The model under review builds one solid part; all positions refer to its coordinate system, in mm. A direction names the side the tool comes from. Coordinates: 2 decimals unless noted, no trailing zeros. Write each loop counter-clockwise with the first axis right and the second up, starting at its lowest first coordinate (ties: lowest second). Pieces come first, ordered by that corner, then holes. Notation, with made-up numbers: (74, 30.25) - (88, 30.25) arc R26 ccw to (88, 60.25) - close; hole circle Ø6 at (-13.75, -11.75). An arc over 180 degrees is marked (long way). Answer as CSV lines item,"result". Start each with the question number.
```python
from build123d import *

# Parameters (mm, degrees)
BOSS_EXTRUDE1_OUTLINE_R = 1.1
BOSS_EXTRUDE1_DEPTH     = 3
BOSS_EXTRUDE2_DEPTH     = 11
BOSS_EXTRUDE3_REACH     = 87.92
SKETCH5_W               = 5
SKETCH5_H               = 2


# Read off the part's stored shape, not the designer's step: Boss-Extrude1
with BuildPart() as part:
    # Boss-Extrude1 outline → Boss-Extrude1 (new body)
    with BuildSketch(Plane.XY):
        with BuildLine():
            Line((-16.861546239, -6.996941033), (-16.235942246, -6.960409413))
            ThreePointArc((-16.235942246, -6.960409413), (-14.264395542, -6.327834493), (-12.678246106, -4.996941033))
            ThreePointArc((-12.678246106, -4.996941033), (13.21501224, 8.679812005), (42.365911354, 5.89781951))
            Line((42.365911354, 5.89781951), (60.907203246, -17.149637471))
            Line((60.907203246, -17.149637471), (78.805808552, -2.750510239))
            Line((78.805808552, -2.750510239), (58.935546262, 21.948902186))
            Line((58.935546262, 21.948902186), (48.942403416, 13.909586673))
            ThreePointArc((48.942403416, 13.909586673), (12.120494673, 18.357071745), (-21.044846371, 1.753058967))
            ThreePointArc((-21.044846371, 1.753058967), (-21.710837424, -3.940345657), (-16.861546239, -6.996941033))
        make_face()
        Polygon((-15.008213446, -0.217369118), (-15.079375496, -0.657391661), (-14.639590345, -0.883380518), (-14.841297197, -1.275911723), (-14.495267888, -1.621941033), (-14.810453449, -1.937126594), (-14.586057014, -2.377726392), (-14.983250587, -2.580016139), (-14.906078059, -3.068407726), (-15.346355155, -3.137977509), (-15.423969348, -3.626299102), (-15.864183346, -3.556331166), (-16.088978162, -3.996727842), (-16.485988624, -3.794078961), (-16.835934444, -4.143392379), (-17.150834826, -3.827921897), (-17.591637385, -4.051919766), (-17.793567832, -3.654543407), (-18.282029013, -3.731274208), (-18.351200586, -3.290934374), (-18.839451787, -3.212878581), (-18.769085755, -2.772728041), (-19.209278949, -2.547535028), (-19.006271099, -2.150708001), (-19.355267888, -1.800446409), (-19.039512742, -1.485831463), (-19.263111863, -1.044826504), (-18.865553043, -0.843255522), (-18.941842054, -0.354725146), (-18.501439842, -0.285951839), (-18.422942512, 0.202228569), (-17.982855791, 0.131464499), (-17.757264764, 0.571453851), (-17.360621498, 0.368087198), (-17.01004442, 0.716767072), (-16.695715168, 0.400727521), (-16.254508168, 0.623927711), (-16.053296817, 0.226186755), (-15.564697645, 0.302033914), (-15.496322662, -0.138430316), align=None, mode=Mode.SUBTRACT)
        with Locations((68.60124446, -8.393050085)):
            Circle(BOSS_EXTRUDE1_OUTLINE_R, mode=Mode.SUBTRACT)
        Polygon((72.402709352, -2.767977433), (62.295668796, -10.898921739), (47.439985558, 7.567198225), (57.547026113, 15.698142531), align=None, mode=Mode.SUBTRACT)
        with Locations((51.208221203, 13.165538506)):
            Circle(BOSS_EXTRUDE1_OUTLINE_R, mode=Mode.SUBTRACT)
    extrude(amount=BOSS_EXTRUDE1_DEPTH)

    # Sketch4 → Boss-Extrude2 (add)
    with BuildSketch(Plane.XY.offset(3)):
        Polygon((13.242665436, 16.771623459), (18.214871239, 17.298092309), (18.372811894, 15.806430568), (13.40060609, 15.279961718), align=None)
        Polygon((13.847221233, 11.061929815), (18.819427036, 11.588398665), (18.661486381, 13.080060406), (13.689280578, 12.553591556), align=None)
    extrude(amount=BOSS_EXTRUDE2_DEPTH)

    # Sketch5 → Boss-Extrude3 (add, up to next)
    with BuildSketch(Plane(origin=(-1.16269721, 10.981029202, 0), x_dir=(0.994441160657232, 0.10529376995196534, 0), z_dir=(-0.10529376995196534, 0.994441160657232, 0)), mode=Mode.PRIVATE) as boss_extrude3_sk1:
        with Locations((17.434999048, -13)):
            Rectangle(SKETCH5_W, SKETCH5_H)
    boss_extrude3_tool1 = extrude(boss_extrude3_sk1.sketch, amount=BOSS_EXTRUDE3_REACH, mode=Mode.PRIVATE) - part.part
    add(boss_extrude3_tool1.solids().sort_by_distance((16.175383, 12.816826, 13))[0])


solid = part.part
```
(1) For faces 1 (the cylindrical face through (-14.29, -6.34, 1.48)), 2 (the flat face through (16.21, 12.82, 7.44)), 3 (the flat face through (16.3, 11.32, 8.42)), 4 (the flat face through (54.972, -1.795, 1.479)), list the 3-axis set-ups (+Z, -Z, +X, -X, +Y, -Y) from which the entire face can be reached by the end or side of a thin tool; tool diameter is ignored.
(2) Add section C-C on x = 1.5. Give the boundary of the cut face in (y, z).
(3) Add section B-B on x = 54. Give the boundary of the cut face in (y, z).
(4) Wall thickness on line 1 (Z direction, x = 3, y = 14.5); line 2 (Y direction, x = 16, z = 7.5); line 3 (Y direction, x = 65, z = 2.5): over which ranges is each line inside the solid? List them lowest first.
(5) For pin 1 (11.5 mm diameter, centred on x = 28.5, y = 6.5, fed in from +Z); pin 2 (8 mm diameter, centred on x = 54.5, y = 18, fed in from -Z); pin 3 (1 mm diameter, centred on y = -0.5, z = 2.5, fed in from +X), all flat-tipped, find the tip position at first contact; note any pin that passes through.
(6) Add section D-D on y = -13. Give the boundary of the cut face in (x, z), then the cut area to 3 significant figures.
(7) Add section A-A on z = 4.5. Give the boundary of the cut face in (x, y), then the cut area to 3 significant figures.
(8) The part is to be moulded in two halves that separate along Z. For faces 5 (the cylindrical face through (69.65, -8.06, 1.48)), 6 (the flat face through (15.922, 15.547, 7.437)), say which applies: released by +Z, released by -Z, zero draft, split by the parting line, or undercut.
Reported:
1,face 1,"+Z, -Z, -Y"
1,face 2,"-X"
1,face 3,"+Z, +X, -Y"
1,face 4,"+Z, -Z"
2,outline,"(4.85, 0) - (15.56, 0) - (15.56, 3) - (4.85, 3) - close"
3,outline,"(-8.56, 0) - (-0.59, 0) - (-0.59, 3) - (-8.56, 3) - close; (12.84, 0) - (17.98, 0) - (17.98, 3) - (12.84, 3) - close"
4,line 1,"0 to 3"
4,line 2,"11.29 to 12.8, 15.56 to 17.06"
4,line 3,"-13.86 to -8.72, 6.43 to 14.41"
5,pin 1,"z = 3"
5,pin 2,"z = 0"
5,pin 3,"x = 77.4"
6,outline,"(57.57, 0) - (66.07, 0) - (66.07, 3) - (57.57, 3) - close"
6,area,"25.5 mm²"
7,outline,"(13.24, 16.77) - (13.4, 15.28) - (18.37, 15.81) - (18.21, 17.3) - close; (13.69, 12.55) - (13.85, 11.06) - (18.82, 11.59) - (18.66, 13.08) - close"
7,area,"15.0 mm²"
8,face 5,"zero draft"
8,face 6,"undercut"
